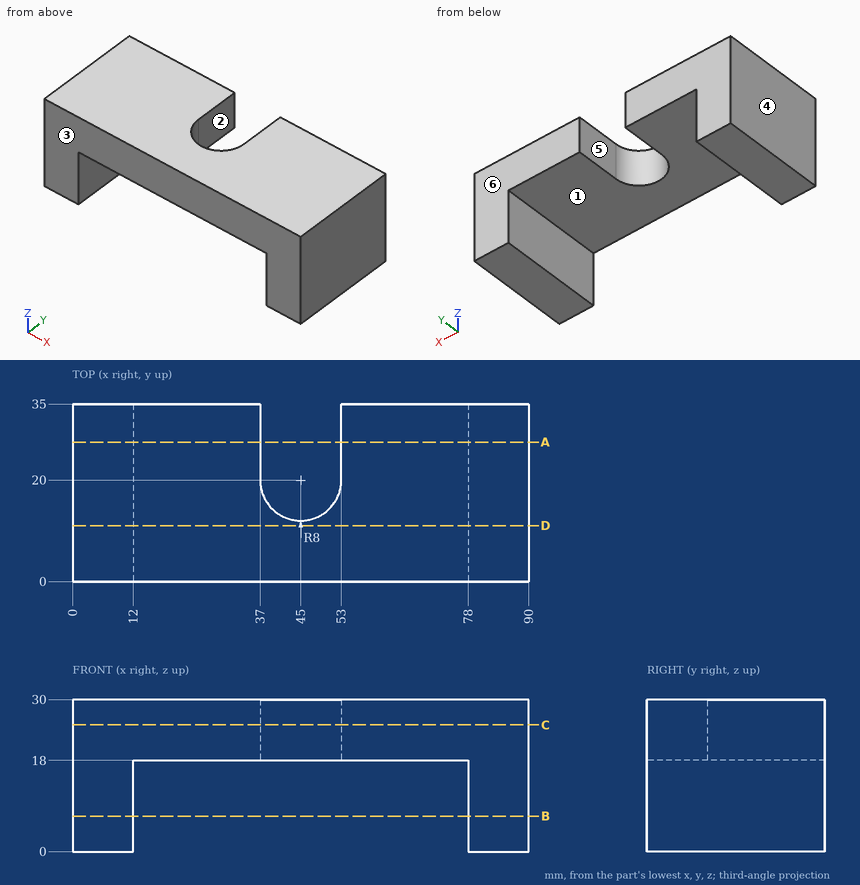
Source: three-view drawing plus pictorial views. Frame: mm from the lowest corner of the part. A direction names the side the tool comes from. Round coordinates to 2 decimals unless told otherwise and drop trailing zeros. Loops run counter-clockwise (first coordinate to the right, second up) from the corner with the lowest first, then second, coordinate; pieces in that order, holes last.
Item 1: Section D-D, the plane y = 11. Output: boundary loops of the cut face in (x, z), plus the area to 3 significant figures.
Checked values:
outline: (0, 0) - (12, 0) - (12, 18) - (78, 18) - (78, 0) - (90, 0) - (90, 30) - (0, 30) - close
area: 1,510 mm2
Item 2: Section A-A, the plane y = 27.5. Output: boundary loops of the cut face in (x, z), plus the area to 3 significant figures.
Checked values:
outline: (0, 0) - (12, 0) - (12, 18) - (37, 18) - (37, 30) - (0, 30) - close; (53, 18) - (78, 18) - (78, 0) - (90, 0) - (90, 30) - (53, 30) - close
area: 1,320 mm2
Item 3: Mould query, pull axis X, two halves, no side actions, for the marked faces 4, 5 and 6. Classes: released by +X, released by -X, zero draft, split by the parting line, or undercut.
Checked values:
face 4: released by -X
face 5: undercut
face 6: zero draft
Item 4: Reachability of the marked faces 1, 2 and 3 from +Z, -Z, +X, -X, +Y, -Y: full face, straight path, thin tool, end or side. Return the list, or none.
Checked values:
face 1: -Z, +Y, -Y
face 2: +Z, -Z, +Y
face 3: +Z, -Z, +X, -X, -Y
Item 5: Section C-C, the plane z = 25. Output: boundary loops of the cut face in (x, y).
Checked values:
outline: (0, 0) - (90, 0) - (90, 35) - (53, 35) - (53, 20) arc R8 cw to (37, 20) - (37, 35) - (0, 35) - close
Item 6: Line query: L1, parallel to X at y = 25.5, z = 3.75; L2, parallel to Z at x = 48, y = 2; L3, parallel to X at y = 13.5, z = 26. Output: solid intervals per line, ascending.
Checked values:
L1: x = 0 to 12, 78 to 90
L2: z = 18 to 30
L3: x = 0 to 40.34, 49.66 to 90
Item 7: Contact query for flat-ended pins moving along their axis: P1, Ø8, axis at x = 18.5, z = 13, coming from the -Y side; P2, Ø12, axis at x = 22, y = 16.5, coming from the -Z side. Output: stop coordinate, or through.
Checked values:
P1: passes through
P2: stops at z = 18
Item 8: Section B-B, the plane z = 7. Output: boundary loops of the cut face in (x, y), plus the area to 3 significant figures.
Checked values:
outline: (0, 0) - (12, 0) - (12, 35) - (0, 35) - close; (78, 0) - (90, 0) - (90, 35) - (78, 35) - close
area: 840 mm2
